Input: part model. Units: mm. Frame: model coordinates. Face numbers are marked on the shaded views. A direction names the side the tool comes from. Round coordinates to 2 decimals unless told otherwise and drop trailing zeros. Loops run counter-clockwise (first coordinate to the right, second up) from the corner with the lowest first, then second, coordinate; pieces in that order, holes last. Notation, with made-up numbers: (82.25, 49.5) - (118.25, 49.5) arc R27 ccw to (118.25, 77.5) - close; hole circle Ø7 at (-39.75, 55.25). An arc over 180 degrees is marked (long way). Write each question's results on one line, items separated by ' | '.
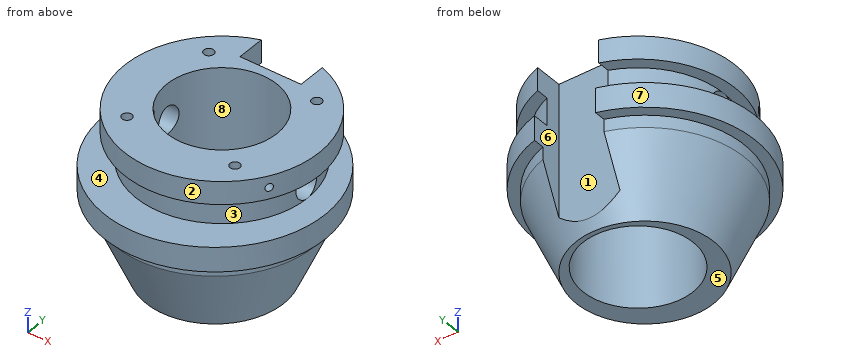
from build123d import *

# Parameters (mm, degrees)
ESQUISSE1_R                  = 36
BASE_EXTRUSION_DEPTH         = 8
ESQUISSE2_R                  = 32.5
BOSS_EXTRU_1_DEPTH           = 4
ESQUISSE4_R                  = 28
BOSS_EXTRU_2_DEPTH           = 9
ESQUISSE5_R                  = 31.8
BOSS_EXTRU_3_DEPTH           = 7.5
ESQUISSE6_R                  = 18
ENL_V_MAT_EXTRU_1_DEPTH      = 52.5
ESQUISSE10_W                 = 20
ESQUISSE10_H                 = 14.61003861
ENL_V_MAT_EXTRU_5_DEPTH      = 52.5
R_P_TITION_CIRCULAIRE1_COUNT = 4
ESQUISSE13_R                 = 4.5
ENL_V_MAT_EXTRU_6_DEPTH      = 37
ENL_V_MAT_EXTRU_6_DEPTH_BACK = 37
ENL_V_START                  = -31.8
ESQUISSE14_R                 = 1.23
ENL_V_MAT_EXTRU_7_DEPTH      = 13.842074
R_P_TITION_CIRCULAIRE2_COUNT = 2
R_P_TITION_CIRCULAIRE2_ANGLE = 120


with BuildPart() as part:
    # Esquisse1 → Base-Extrusion (new body)
    with BuildSketch(Plane.XY):
        Circle(ESQUISSE1_R)
    extrude(amount=BASE_EXTRUSION_DEPTH)

    # Esquisse2 → Boss.-Extru.1 (add)
    with BuildSketch(Plane(origin=(0, 0, 0), x_dir=(-1, 0, 0), z_dir=(0, 0, -1))):
        Circle(ESQUISSE2_R)
    extrude(amount=BOSS_EXTRU_1_DEPTH)

    # Esquisse3 → Boss.-Révol.1 (revolve)
    with BuildSketch(Plane(origin=(0, 0, 0), x_dir=(0, 0, -1), z_dir=(1, 0, 0))):
        Polygon((4, 32.5), (27, 22.499315376), (27, 0), (4, 0), align=None)
    revolve(axis=Axis((0, 0, 0), (0, 0, -1)))

    # Esquisse4 → Boss.-Extru.2 (add)
    with BuildSketch(Plane.XY.offset(8)):
        with Locations((0, 3)):
            Circle(ESQUISSE4_R)
    extrude(amount=BOSS_EXTRU_2_DEPTH)

    # Esquisse5 → Boss.-Extru.3 (add)
    with BuildSketch(Plane.XY.offset(17)):
        with Locations((0, 3)):
            Circle(ESQUISSE5_R)
    extrude(amount=BOSS_EXTRU_3_DEPTH)

    # Esquisse6 → Enlèv. mat.-Extru.1 (cut, through all)
    with BuildSketch(Plane.XY.offset(24.5)):
        with Locations((0, 3)):
            Circle(ESQUISSE6_R)
    extrude(amount=-ENL_V_MAT_EXTRU_1_DEPTH, mode=Mode.SUBTRACT)

    # Esquisse10 → Enlèv. mat.-Extru.5 (cut, through all)
    with BuildSketch(Plane.XY.offset(24.5)):
        with Locations((0, 31.305019305)):
            Rectangle(ESQUISSE10_W, ESQUISSE10_H)
    extrude(amount=-ENL_V_MAT_EXTRU_5_DEPTH, mode=Mode.SUBTRACT)

    # Esquisse11 → Perçage1 (revolve, cut)
    with BuildSketch(Plane(origin=(-17.67766953, 20.67766953, 24.5), x_dir=(0, -1, 0), z_dir=(1, 0, 0))):
        Polygon((0, 0), (0, 12.976398506), (1.625, 12), (1.625, 0), align=None)
    per_age1 = revolve(axis=Axis((-17.67766953, 20.67766953, 28.744199587), (0, 0, -1)), mode=Mode.SUBTRACT)

    # Répétition circulaire1: Perçage1 ×4 about axis
    r_p_tition_circulaire1_axis = Axis((0, 3, 0), (0, 0, 1))
    for i in range(1, R_P_TITION_CIRCULAIRE1_COUNT):
        add(per_age1.rotate(r_p_tition_circulaire1_axis, i * 360 / R_P_TITION_CIRCULAIRE1_COUNT), mode=Mode.SUBTRACT)

    # Esquisse13 → Enlèv. mat.-Extru.6 (cut, two sides)
    with BuildSketch(Plane(origin=(0, 0, 0), x_dir=(0, 0, -1), z_dir=(1, 0, 0))) as enl_v_mat_extru_6_sk:
        with Locations((-12.5, 3)):
            Circle(ESQUISSE13_R)
    extrude(amount=ENL_V_MAT_EXTRU_6_DEPTH, mode=Mode.SUBTRACT)
    extrude(enl_v_mat_extru_6_sk.sketch, amount=-ENL_V_MAT_EXTRU_6_DEPTH_BACK, mode=Mode.SUBTRACT)

    # Esquisse14 → Enlèv. mat.-Extru.7 (cut)
    with BuildSketch(Plane(origin=(-1.299038106, 0.75, 0), x_dir=(0, 0, 1), z_dir=(-0.866025404, 0.5, 0)).offset(ENL_V_START)):
        with Locations((20.75, 2.598076211)):
            Circle(ESQUISSE14_R)
    enl_v_mat_extru_7 = extrude(amount=ENL_V_MAT_EXTRU_7_DEPTH, mode=Mode.SUBTRACT)

    # Répétition circulaire2: Enlèv. mat.-Extru.7 ×2 about axis
    r_p_tition_circulaire2_axis = Axis((0, 3, 0), (0, 0, -1))
    for i in range(1, R_P_TITION_CIRCULAIRE2_COUNT):
        add(enl_v_mat_extru_7.rotate(r_p_tition_circulaire2_axis, i * R_P_TITION_CIRCULAIRE2_ANGLE / (R_P_TITION_CIRCULAIRE2_COUNT - 1)), mode=Mode.SUBTRACT)


solid = part.part
1. Section query B-B, the plane y = 0. Count the separate pieces of the cut face and the enclosed holes in it, plus the area to 3 significant figures.
Answer:
separate pieces: 4 | enclosed holes: 0 | area: 1,110 mm^2
2. Line query: line 1 (Y direction, x = 0, z = 14); line 2 (Z direction, x = 20.25, y = 3); line 3 (Z direction, x = -27, y = -19). Output: solid intervals per line, ascending. Write a range as [from, to].
Answer:
line 1: [-25, -15], [21, 24] | line 2: [-27, 8], [17, 24.5] | line 3: [0, 8]
3. Section query C-C, the plane z = -11.5. Output: boundary loops of the cut face in (x, y).
Answer:
outline: (-10, 24) - (-10, 27.48) arc R29.24 ccw (long way) to (10, 27.48) - (10, 24) - close; hole circle Ø36 at (0, 3)
4. Set-up query: the marked faces 1, 2, 3 and 4. Return all of +Z, -Z, +X, -X, +Y, -Y with unobstructed straight access to the full face (end or side cutting, diameter ignored); none if empty.
Answer:
face 1: +Z, -Z, +Y | face 2: +Z | face 3: -Y | face 4: none
5. Section query A-A, the plane x = 0. Output: boundary loops of the cut face in (y, z).
Answer:
outline: (-36, 0) - (-32.5, 0) - (-32.5, -4) - (-22.5, -27) - (-15, -27) - (-15, 24.5) - (-28.8, 24.5) - (-28.8, 17) - (-25, 17) - (-25, 8) - (-36, 8) - close; (21, -27) - (22.5, -27) - (24, -23.55) - (24, 24.5) - (21, 24.5) - close
6. Mould query, pull axis X, two halves, no side actions, for the marked faces 5, 6, 7 and 8. Classes: pulls with the +X half, pulls with the -X half, needs draft (parallel to the pull), parting line crosses it, or undercut.
Answer:
face 5: needs draft | face 6: undercut | face 7: parting line crosses it | face 8: undercut
7. Contact query for flat-ended pins moving along their axis: pin 1 (5 mm diameter, centred on x = -17.68, y = 20.68, fed in from -Z); pin 2 (8 mm diameter, centred on y = -2.5, z = -5.5, fed in from +X); pin 3 (10 mm diameter, centred on x = 26, z = -21.5, fed in from +Y); pin 4 (4 mm diameter, centred on x = -17.68, y = -14.68, fed in from -Z). Output: stop coordinate, or through.
Answer:
pin 1: z = -21.92 | pin 2: x = 32.5 | pin 3: y = 14.33 | pin 4: z = -27
8. Section query D-D, the plane z = -6. Output: boundary loops of the cut face in (x, y).
Answer:
outline: (-10, 24) - (-10, 30.01) arc R31.63 ccw (long way) to (10, 30.01) - (10, 24) - close; hole circle Ø36 at (0, 3)
